Geometry: final body of the model. Coordinates: model frame, mm. Face numbers are marked on the shaded views. A direction names the side the tool comes from. Coordinates: 2 decimals unless noted, no trailing zeros. Loops run counter-clockwise (first coordinate to the right, second up) from the corner with the lowest first, then second, coordinate; pieces in that order, holes last. Notation, with made-up numbers: (-11, 24) - (11, 24) arc R22 cw to (11, 32) - close; hole circle Ø7 at (1.25, 82). An arc over 180 degrees is marked (long way). Put each result on its own line as item: value. Start each with the question number.
1) Section D-D on y = 12. Output: boundary loops of the cut face in (x, z), and give its area (3 significant figures).
2) Section C-C on x = 93.5. Output: boundary loops of the cut face in (y, z), and give its area (3 significant figures).
3) Reachability of the marked faces 1 and 2 from +Z, -Z, +X, -X, +Y, -Y: full face, straight path, thin tool, end or side. Return the list, or none.
4) Section A-A on x = 65. Output: boundary loops of the cut face in (y, z).
5) Draft query along Y for the marked faces 3, 4 and 5. Return one class per face: +Y half, -Y half, draft (parallel to the pull), parting line (faces both ways), or undercut.
6) Section B-B on z = 5.5. Output: boundary loops of the cut face in (x, y).
7) Contact query for flat-ended pins moving along their axis: pin 1 Ø2 at (x, y) = (24, 64.5) entering from -Z; pin 2 Ø1.5 at (x, z) = (79.5, 6) entering from +Y; pin 3 Ø6.5 at (x, y) = (47, 26.5) entering from +Z; pin 4 Ø2 at (x, z) = (66.5, 6) entering from +Y. Output: stop coordinate, or through.
8) Material intervals for line 1 along Y through (x, z) = (45, 1); line 2 along Y through (x, z) = (44.5, 0.75); line 3 along X through (y, z) = (71.5, 4.25), sorted ascending. Write a range as from..to.
```python
from build123d import *

# Parameters (mm, degrees)
SKETCH_R        = 50
PAD_DEPTH       = 7
POCKET_DEPTH    = 7.001
SKETCH005_W     = 30
SKETCH005_H     = 7
POCKET001_DEPTH = 3
SKETCH030_R     = 3
POCKET022_DEPTH = 15


with BuildPart() as part:
    # Sketch → Pad (new body)
    with BuildSketch(Plane.XY):
        with Locations((54.312531, 53.68195)):
            Circle(SKETCH_R)
    extrude(amount=PAD_DEPTH)

    # Sketch004 (on Face3 of Pad) → Pocket (cut, through all)
    with BuildSketch(Plane.XY.offset(7)):
        Polygon((56.333257, 35.748194), (68.833257, 57.398829), (68.833257, 64.398829), (43.833257, 64.398829), (37.771079, 60.898829), (50.271079, 39.248194), align=None)
    extrude(amount=-POCKET_DEPTH, mode=Mode.SUBTRACT)

    # Sketch005 (on Face3 of Pocket) → Pocket001 (cut)
    with BuildSketch(Plane.XY.offset(7)):
        with Locations((83.833257, 60.898829)):
            Rectangle(SKETCH005_W, SKETCH005_H)
        Polygon((56.333257, 35.748194), (41.333257, 9.767432), (35.271079, 13.267432), (50.271079, 39.248194), align=None)
        Polygon((37.771079, 60.898829), (22.771079, 86.879591), (28.833257, 90.379591), (43.833257, 64.398829), align=None)
    extrude(amount=-POCKET001_DEPTH, mode=Mode.SUBTRACT)

    # Sketch030 (on Face3 of Pocket001) → Pocket022 (cut)
    with BuildSketch(Plane.XY.offset(7)):
        with Locations((45.802168, 24.507813)):
            Circle(SKETCH030_R)
        with Locations((33.302168, 75.63921)):
            Circle(SKETCH030_R)
        with Locations((83.833257, 60.898829)):
            Circle(SKETCH030_R)
    extrude(amount=-POCKET022_DEPTH, mode=Mode.SUBTRACT)


solid = part.part
```
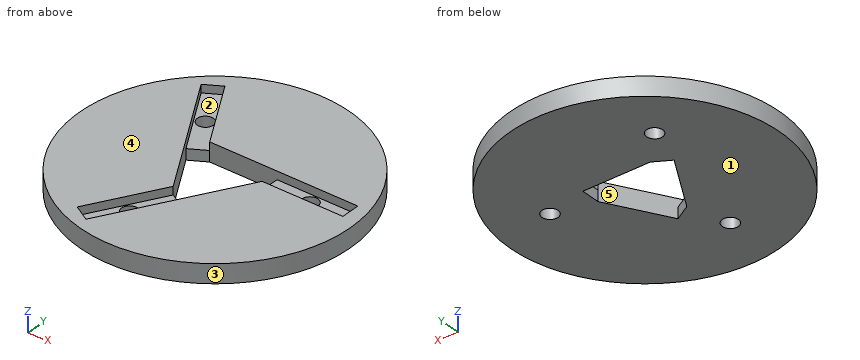
Answer block:
1. outline: (26.7, 0) - (81.93, 0) - (81.93, 7) - (42.62, 7) - (42.62, 4) - (37.47, 4) - (37.47, 7) - (26.7, 7) - close
1. area: 371 mm²
2. outline: (22.63, 0) - (84.74, 0) - (84.74, 7) - (64.4, 7) - (64.4, 4) - (57.4, 4) - (57.4, 7) - (22.63, 7) - close
2. area: 414 mm²
3. face 1: -Z, +X, -X, +Y, -Y
3. face 2: +Z
4. outline: (4.84, 0) - (50.76, 0) - (50.76, 7) - (4.84, 7) - close; (64.4, 0) - (102.53, 0) - (102.53, 7) - (64.4, 7) - close
5. face 3: parting line
5. face 4: draft
5. face 5: undercut
6. outline: circle Ø100 at (54.31, 53.68); hole (22.77, 86.88) - (50.27, 39.25) - (35.27, 13.27) - (41.33, 9.77) - (68.83, 57.4) - (98.83, 57.4) - (98.83, 64.4) - (43.83, 64.4) - (28.83, 90.38) - close
7. pin 1: stops at z = 0
7. pin 2: stops at y = 97.3
7. pin 3: stops at z = 4
7. pin 4: stops at y = 102.41
8. line 1: y = 4.56..21.62, 27.4..48.38, 64.4..102.81
8. line 2: y = 4.65..21.81, 27.21..49.24, 64.4..102.71
8. line 3: x = 7.6..31.65, 39.73..101.03
